The listing builds one solid part. Answer for the finished solid, in the listing's coordinates (mm). A direction names the side the tool comes from. Give positions to 0.01 mm unless a question says otherwise; leave off trailing zeros. Loops run counter-clockwise (first coordinate to the right, second up) from the corner with the lowest first, then second, coordinate; pieces in that order, holes last.
Item 1: Section B-B, the plane x = -169.5 is taken. Give the vertices of the cut face in (y, z).
Item 2: Section C-C, the plane z = 218.5 is taken. Give the vertices of the cut face in (x, y), and give its area (3 significant figures).
Item 3: Section D-D, the plane y = -4 is taken. Give the vertices of the cut face in (x, z).
Item 4: A tool of negligible diameter and unlimited length cuts with its end or side. For faces 1 (the face through (-198.51, -18.08, 230.84)), 2 (the face through (-206.231, -11.832, 206.457)), 3 (the face through (-150, -24, 125)), from which of +Z, -Z, +X, -X, +Y, -Y can it reach the whole face along a straight path? Write none if from no direction.
Item 5: Consider line 1 along Z through (x, y) = (-149.5, -17.25); line 2 along X through (y, z) = (-14.25, 239.5); line 3 along X through (y, z) = (-17.5, 231). Determine where each line is inside the solid, lowest interval first.
Item 6: Section A-A, the plane x = -212 is taken. Give the vertices of the cut face in (y, z), and give its area (3 significant figures).
Item 7: Each of these flat-tipped pins is pushed along its axis until it touches: pin 1 Ø9.5 at (x, y) = (-162.5, -20.5) entering from +Z; pin 2 Ø5 at (x, z) = (-124, 121) entering from -Y; pin 3 Ø13 at (x, y) = (-162, -19.5) entering from -Z. Where does it stop, or does it pass through?
from build123d import *

# Parameters (mm, degrees)
F1_DEPTH    = 24
F2_R        = 50
F3_T1_DEPTH = 105.7731172378
F3_T3_DEPTH = 66.3378383392
F3_T6_ANGLE = 65.4740658064
F6_DEPTH    = 12
F8_DEPTH    = 12
F9_DEPTH    = 12
F11_DEPTH   = 12


# Not quite as in the source:
# - a fillet or chamfer that OpenCascade refuses, or shapes differently, is made with other operations: its cross-section is extruded or revolved along the edge and cut away or added


with BuildPart() as f1:
    # F0 (on Front) → F1 (new body)
    with BuildSketch(Plane.XZ):
        Polygon((-81.055521965, 64.9488791823), (-7.5541026236, 85.0398655279), (-114.0252747561, 191.5110376604), (-234.0252747561, 191.5110376604), (-240.9712018628, 152.1187275399), (-150.2916823338, 119.1140815738), (-86.9572677666, 28.6631636514), align=None)
    extrude(amount=F1_DEPTH)

    # F2
    f2_edges = [f1.edges().sort_by_distance(p)[0] for p in [
        (-81.055522, -12, 64.948879),
    ]]
    fillet(f2_edges, radius=F2_R)

    # F3: chamfer of 24 on 2 edges, made by hand

    # F3_s2 → F3_t1 (cut)
    with BuildSketch(Plane(origin=(-27.8938692058, 0, -7.6245513401), x_dir=(0, 1, 0), z_dir=(0.9646132681, 0, 0.2636688131))):
        Polygon((0, 108.0223638788), (-24, 84.0223638788), (0, 84.0223638788), align=None)
    extrude(amount=F3_T1_DEPTH, mode=Mode.SUBTRACT)

    # F3_s4 → F3_t3 (cut)
    with BuildSketch(Plane(origin=(-7.6076630021, 0, -46.7742096713), x_dir=(0, 1, 0), z_dir=(0.1605369785, 0, 0.9870298266))):
        Polygon((-24, 90.4309146097), (0, 114.4309146097), (0, 90.4309146097), align=None)
    extrude(amount=F3_T3_DEPTH, mode=Mode.SUBTRACT)

    # F3_s5 → F3_t6 (revolve, cut)
    with BuildSketch(Plane(origin=(3.0420131267, 0, 18.7032153992), x_dir=(0, 1, 0), z_dir=(-0.1605369785, 0, -0.9870298266))):
        Polygon((0, -114.4309146097), (-24, -90.4309146097), (0, -90.4309146097), align=None)
    revolve(axis=Axis((-36.8645055082, 0, 25.1938722697), (0, 1, 0)), revolution_arc=F3_T6_ANGLE, mode=Mode.SUBTRACT)

    # F5 (on face) → F6 (join)
    with BuildSketch(Plane(origin=(0, 0, 0), x_dir=(-1, 0, 0), z_dir=(0, 1, 0))):
        Polygon((84.0423926711, 139.9491429329), (163.5881303991, 155.6373062127), (219.1278844576, 221.8270076437), (193.4163800701, 252.4687853684), (98.1535856538, 197.4687853684), align=None)
    extrude(amount=-F6_DEPTH)

    # F7 (on face) → F8 (cut)
    with BuildSketch(Plane.XZ.offset(24)):
        with BuildLine():
            Line((-143.908641448, 127.432622412), (-100.3174393188, 65.1779339797))
            ThreePointArc((-100.3174393188, 65.1779339797), (-81.5137230154, 85.4553639206), (-56.6396664901, 97.5398673775))
            Line((-56.6396664901, 97.5398673775), (-39.014051648, 102.3576789286))
            Line((-39.014051648, 102.3576789286), (-118.1674103798, 181.5110376604))
            Line((-118.1674103798, 181.5110376604), (-225.6342784443, 181.5110376604))
            Line((-225.6342784443, 181.5110376604), (-229.6660431143, 158.6457639866))
            Line((-229.6660431143, 158.6457639866), (-143.908641448, 127.432622412))
        make_face()
    extrude(amount=-F8_DEPTH, mode=Mode.SUBTRACT)

    # F9 (add): a face of the model
    f9_faces = [f1.faces().sort_by_distance(p)[0] for p in [
        (-164.1324178165, -12, 212.498446066),
    ]]
    extrude(f9_faces, amount=F9_DEPTH)

    # F10 (on face) → F11 (cut)
    with BuildSketch(Plane.XZ.offset(24)):
        Polygon((-104.7010093218, 182.1867722261), (-106.848922609, 190.9420351164), (-191.149564101, 239.6130331747), (-206.0738115642, 221.8270076437), (-180.6356923325, 191.5110376604), (-114.0252747561, 191.5110376604), align=None)
    extrude(amount=-F11_DEPTH, mode=Mode.SUBTRACT)


solid = f1.part
Worked answers:
1. outline: (-24, 126.11) - (0, 126.11) - (0, 238.66) - (-24, 238.66) - (-24, 227.11) - (-12, 227.11) - (-12, 191.51) - (-24, 191.51) - (-24, 181.51) - (-12, 181.51) - (-12, 136.75) - (-24, 136.75) - close
2. outline: (-216.34, -24) - (-203.28, -24) - (-203.28, -12) - (-154.58, -12) - (-154.58, -24) - (-134.58, -24) - (-134.58, 0) - (-216.34, 0) - close
2. area: 1,380 mm2
3. outline: (-240.97, 152.12) - (-150.29, 119.11) - (-102.17, 50.39) arc R70 cw to (-55.32, 92.72) - (-23.84, 101.32) - (-91.06, 168.54) - (-98.15, 197.47) - (-193.42, 252.47) - (-219.13, 221.83) - (-193.69, 191.51) - (-234.03, 191.51) - close
4. face 1: -Y
4. face 2: -X, +Y, -Y
4. face 3: +Z, -Z, +X, -X, -Y
5. line 1: z = 117.98 to 129.47, 181.51 to 191.51, 215.57 to 227.11
5. line 2: x = -204.3 to -191.24, -190.95 to -170.95
5. line 3: x = -211.43 to -198.38, -176.23 to -156.23
6. outline: (-24, 141.57) - (0, 141.57) - (0, 191.51) - (-24, 191.51) - (-24, 181.51) - (-12, 181.51) - (-12, 152.22) - (-24, 152.22) - close; (-24, 213.33) - (0, 213.33) - (0, 230.32) - (-24, 230.32) - close
6. area: 1,250 mm2
7. pin 1: stops at z = 237.36
7. pin 2: stops at y = -12
7. pin 3: stops at z = 121.01
